For this review, use the dimensioned drawing (mm, ordinates from the lowest corner) and the shaded views. Round coordinates to 2 decimals unless told otherwise and drop trailing zeros. Order: outer loops, then holes, each group sorted by start corner. A loop starts at its lowest first (then second) coordinate and runs counter-clockwise, first axis right, second up. Notation, with made-up numbers: (4.5, 16) - (46.5, 16) arc R21 cw to (46.5, 55) - close; hole circle Ø1 at (15, -6.5). An arc over 180 degrees is marked (long way). Write item = value, one per line.
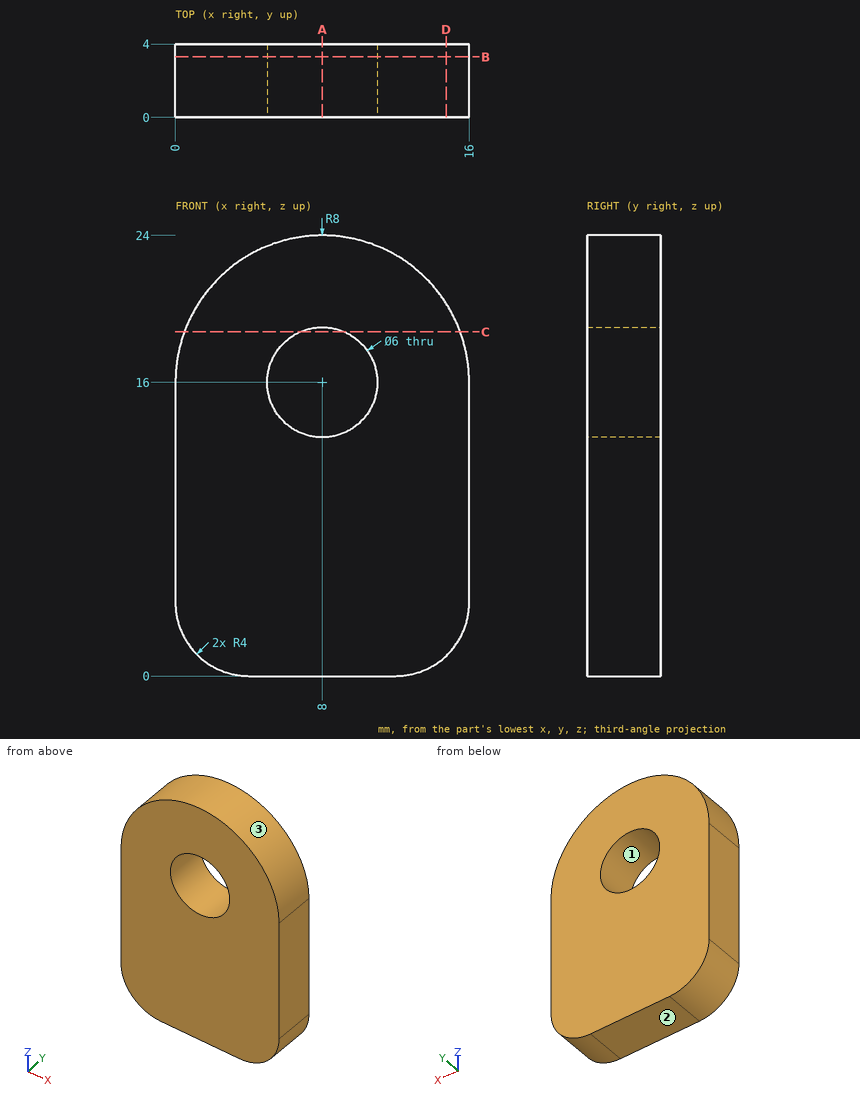
Item 1: Take a section at C-C, the plane z = 18.75. State the section outline as (x, y) points.
Data:
outline = (0.49, 0) - (6.8, 0) - (6.8, 4) - (0.49, 4) - close; (9.2, 0) - (15.51, 0) - (15.51, 4) - (9.2, 4) - close
Item 2: Take a section at D-D, the plane x = 14.75. State the section outline as (y, z) points.
Data:
outline = (0, 1.1) - (4, 1.1) - (4, 20.29) - (0, 20.29) - close
Item 3: For line 1 along X through (y, z) = (1.45, 16); line 2 along Z through (x, y) = (5.5, 1.45); line 3 along Z through (x, y) = (7, 0.4), list the stretches that pass through material, from the lowest coordinate up. Write a range as [from, to].
Data:
line_1 = [0, 5], [11, 16]
line_2 = [0, 14.34], [17.66, 23.6]
line_3 = [0, 13.17], [18.83, 23.94]
Item 4: Take a section at A-A, the plane x = 8. State the section outline as (y, z) points, and give its area (3 significant figures).
Data:
outline = (0, 0) - (4, 0) - (4, 13) - (0, 13) - close; (0, 19) - (4, 19) - (4, 24) - (0, 24) - close
area = 72.0 mm2
Item 5: The part is to be moulded in two halves that separate along Z. For the marked faces 1, 2 and 3, say which applies: +Z half, -Z half, draft (parallel to the pull), parting line (faces both ways), or undercut.
Data:
face_1 = undercut
face_2 = -Z half
face_3 = +Z half
Item 6: Take a section at B-B, the plane y = 3.3. State the section outline as (x, z) points, and give its area (3 significant figures).
Data:
outline = (0, 4) arc R4 ccw to (4, 0) - (12, 0) arc R4 ccw to (16, 4) - (16, 16) arc R8 ccw to (0, 16) - close; hole circle Ø6 at (8, 16)
area = 321 mm2
Item 7: Insertion check: P1, Ø1, axis at x = 12, y = 3.5, coming from the +Z side. The pin has a flat end and moves straight along its axis. Give the tip position at first contact, or say it passes through.
Data:
P1 = 23.19
